Here's how the part is built. I have some questions about the finished solid (model axes, mm). Face numbers are marked on the shaded views. A direction names the side the tool comes from. Coordinates: 2 decimals unless noted, no trailing zeros. Write each loop counter-clockwise with the first axis right and the second up, starting at its lowest first coordinate (ties: lowest second). Pieces come first, ordered by that corner, then holes. Notation, with made-up numbers: (23, 27) - (56, 27) arc R17 cw to (56, 43) - close; hole circle Ø8 at (5, 9). An arc over 180 degrees is marked (long way). Answer in a Markdown table with one row per item. Add a question column.
Item 1: Imagine slicing it at C-C (z = 31). Please give me the cut outline in (x, y), plus the area to 3 significant figures.
Item 2: Which directions (+Z, -Z, +X, -X, +Y, -Y) give clear straight access to the entire face, cutting with the end or side of a thin tool? Please do the marked faces 1, 2 and 3.
Item 3: I'm going to push flat-ended pins straight in: pin 1 (3.5 mm diameter, centred on x = -5, z = -11, fed in from +Y); pin 2 (5 mm diameter, centred on y = 9, z = 11, fed in from -X); pin 3 (3.5 mm diameter, centred on x = -36, z = 48, fed in from +Y). Where does each tip first touch, or does it pass through?
Item 4: Imagine slicing it at A-A (x = -40.5). Please give me the cut outline in (y, z), plus the area to 3 significant figures.
Item 5: If I drill on probe 1 along Z at (x, y) = (-39.5, 8); probe 2 along X at (y, z) = (24.25, 37); probe 3 along X at (y, z) = (10.25, -45), over which ranges is the centre line in solid material (lowest first)? Write a range as from..to.
Item 6: We'd pull the mould along X, two halves only. Please class the marked faces 4, 5 and 6: +X half, -X half, draft (parallel to the pull), parting line (faces both ways), or undercut.
Item 7: Imagine slicing it at D-D (x = 47). Please give me the cut outline in (y, z), plus the area to 3 significant figures.
Item 8: Imagine slicing it at B-B (z = 46). Please give me the cut outline in (x, y), plus the area to 3 significant figures.
from build123d import *

# Parameters (mm, degrees)
BOSS_EXTRUDE1_DEPTH      = 2.5
BOSS_EXTRUDE1_DEPTH_BACK = 5
SKETCH3_W                = 7
SKETCH3_H                = 22
BOSS_EXTRUDE4_DEPTH      = 2.5
BOSS_EXTRUDE5_DEPTH      = 20
SKETCH7_R                = 3.75
BOSS_EXTRUDE6_DEPTH      = 5.5
SKETCH10_R               = 1.05
CUT_EXTRUDE1_DEPTH       = 2.5
SKETCH14_W               = 125
SKETCH14_H               = 7.5
SKETCH14_W_2             = 18
SKETCH14_H_2             = 1.5
BOSS_EXTRUDE8_DEPTH      = 10
SKETCH15_W               = 2.2
SKETCH15_H               = 17.5
SKETCH15_W_2             = 2.5
BOSS_EXTRUDE9_DEPTH      = 10
SKETCH16_R               = 1.4
CUT_EXTRUDE3_DEPTH       = 114
SKETCH17_W               = 7
SKETCH17_H               = 30
BOSS_EXTRUDE10_DEPTH     = 70
SKETCH18_W               = 45.75
SKETCH18_H               = 7.5
BOSS_EXTRUDE11_DEPTH     = 10


with BuildPart() as part:
    # Sketch2 → Boss-Extrude1 (new, two sides: drawn at the far end of the back side and taken through both)
    with BuildSketch(Plane(origin=(0, 0, 0), x_dir=(1, 0, 0), z_dir=(0, 1, 0)).offset(-BOSS_EXTRUDE1_DEPTH_BACK)):
        with BuildLine():
            Line((62.5, 25), (62.5, -25))
            ThreePointArc((62.5, -25), (53.127416998, -47.627416998), (30.5, -57))
            Line((30.5, -57), (23.5, -57))
            Line((23.5, -57), (23.5, -35))
            Line((23.5, -35), (30.5, -35))
            ThreePointArc((30.5, -35), (40.5, -25), (30.5, -15))
            Line((30.5, -15), (-38.5, -15))
            ThreePointArc((-38.5, -15), (-48.5, -25), (-38.5, -35))
            Line((-38.5, -35), (-31.5, -35))
            Line((-31.5, -35), (-31.5, -57))
            Line((-31.5, -57), (-38.5, -57))
            Line((-38.5, -57), (-62.5, -57))
            Line((-62.5, -57), (-62.5, 57))
            Line((-62.5, 57), (-38.5, 57))
            Line((-38.5, 57), (-31.5, 57))
            Line((-31.5, 57), (-31.5, 35))
            Line((-31.5, 35), (-38.5, 35))
            ThreePointArc((-38.5, 35), (-48.5, 25), (-38.5, 15))
            Line((-38.5, 15), (30.5, 15))
            ThreePointArc((30.5, 15), (40.5, 25), (30.5, 35))
            Line((30.5, 35), (23.5, 35))
            Line((23.5, 35), (23.5, 57))
            Line((23.5, 57), (30.5, 57))
            ThreePointArc((30.5, 57), (53.127416998, 47.627416998), (62.5, 25))
        make_face()
    extrude(amount=BOSS_EXTRUDE1_DEPTH + BOSS_EXTRUDE1_DEPTH_BACK)

    # Sketch3 → Boss-Extrude4 (add)
    with BuildSketch(Plane(origin=(0, 2.5, 0), x_dir=(1, 0, 0), z_dir=(0, 1, 0))):
        with Locations((-35, -46)):
            Rectangle(SKETCH3_W, SKETCH3_H)
        with Locations((27, -46)):
            Rectangle(SKETCH3_W, SKETCH3_H)
        with Locations((27, 46)):
            Rectangle(SKETCH3_W, SKETCH3_H)
        with Locations((-35, 46)):
            Rectangle(SKETCH3_W, SKETCH3_H)
    extrude(amount=BOSS_EXTRUDE4_DEPTH)

    # Sketch6 → Boss-Extrude5 (add)
    with BuildSketch(Plane(origin=(0, 5, 0), x_dir=(1, 0, 0), z_dir=(0, 1, 0))):
        Polygon((-38.5, -35), (-31.5, -35), (-31.5, -57), (-38.5, -57), (-38.5, -54.5), (-34, -54.5), (-34, -37.5), (-38.5, -37.5), align=None)
        Polygon((30.5, -35), (23.5, -35), (23.5, -57), (30.5, -57), (30.5, -54.5), (26, -54.5), (26, -37.5), (30.5, -37.5), align=None)
        Polygon((30.5, 37.5), (30.5, 35), (23.5, 35), (23.5, 57), (30.5, 57), (30.5, 54.5), (26, 54.5), (26, 37.5), align=None)
        Polygon((-38.5, 37.5), (-38.5, 35), (-31.5, 35), (-31.5, 57), (-38.5, 57), (-38.5, 54.5), (-34, 54.5), (-34, 37.5), align=None)
    extrude(amount=BOSS_EXTRUDE5_DEPTH)

    # Sketch7 → Boss-Extrude6 (add)
    with BuildSketch(Plane.ZY.offset(-23.5)):
        with Locations((46, 13.75)):
            Circle(SKETCH7_R)
        with Locations(Location((-46, 13.75, 0), (0, 0, 180))):
            Circle(SKETCH7_R)
    extrude(amount=BOSS_EXTRUDE6_DEPTH)

    # Sketch10 → Cut-Extrude1 (cut)
    with BuildSketch(Plane(origin=(-31.5, 0, 0), x_dir=(0, 0, -1), z_dir=(1, 0, 0))):
        with Locations((-42.5, 22)):
            Circle(SKETCH10_R)
        with Locations(Location((-49.5, 22, 0), (0, 0, 180))):
            Circle(SKETCH10_R)
        with Locations((-49.5, 8)):
            Circle(SKETCH10_R)
        with Locations(Location((-42.5, 8, 0), (0, 0, 180))):
            Circle(SKETCH10_R)
        with Locations((42.5, 8)):
            Circle(SKETCH10_R)
        with Locations(Location((49.5, 8, 0), (0, 0, 180))):
            Circle(SKETCH10_R)
        with Locations((49.5, 22)):
            Circle(SKETCH10_R)
        with Locations(Location((42.5, 22, 0), (0, 0, 180))):
            Circle(SKETCH10_R)
    extrude(amount=-CUT_EXTRUDE1_DEPTH, mode=Mode.SUBTRACT)

    # Sketch14 → Boss-Extrude8 (add)
    with BuildSketch(Plane(origin=(0, 2.5, 0), x_dir=(1, 0, 0), z_dir=(0, 1, 0))):
        Rectangle(SKETCH14_W, SKETCH14_H)
        Polygon((-56.5, -49.5), (-62.5, -49.5), (-62.5, -57), (-56.5, -57), (-56.5, -55.5), align=None)
        with Locations((-47.5, -56.25)):
            Rectangle(SKETCH14_W_2, SKETCH14_H_2)
        Polygon((-62.5, 57), (-62.5, 49.5), (-56.5, 49.5), (-56.5, 55.5), (-56.5, 57), align=None)
        with Locations((-47.5, 56.25)):
            Rectangle(SKETCH14_W_2, SKETCH14_H_2)
    extrude(amount=BOSS_EXTRUDE8_DEPTH)

    # Sketch15 → Boss-Extrude9 (add)
    with BuildSketch(Plane.ZY.offset(62.5)):
        with Locations((0, 3.75)):
            Rectangle(SKETCH15_W, SKETCH15_H)
        with Locations((55.75, 3.75)):
            Rectangle(SKETCH15_W_2, SKETCH15_H)
        with Locations((50.75, 3.75)):
            Rectangle(SKETCH15_W_2, SKETCH15_H)
        with Locations((-50.75, 3.75)):
            Rectangle(SKETCH15_W_2, SKETCH15_H)
        with Locations((-55.75, 3.75)):
            Rectangle(SKETCH15_W_2, SKETCH15_H)
    extrude(amount=BOSS_EXTRUDE9_DEPTH)

    # Sketch16 → Cut-Extrude3 (cut)
    with BuildSketch(Plane.XY.offset(57)):
        with Locations((-67.5, 7.25)):
            Circle(SKETCH16_R)
        with Locations((-67.5, 0.25)):
            Circle(SKETCH16_R)
    extrude(amount=-CUT_EXTRUDE3_DEPTH, mode=Mode.SUBTRACT)

    # Sketch17 → Boss-Extrude10 (add)
    with BuildSketch(Plane.XY.offset(-35)):
        with Locations((-35, 10)):
            Rectangle(SKETCH17_W, SKETCH17_H)
        with Locations((27, 10)):
            Rectangle(SKETCH17_W, SKETCH17_H)
    extrude(amount=BOSS_EXTRUDE10_DEPTH)

    # Sketch18 → Boss-Extrude11 (add)
    with BuildSketch(Plane.ZY.offset(62.5)):
        with Locations((-26.625, -1.25)):
            Rectangle(SKETCH18_W, SKETCH18_H)
        with Locations((26.625, -1.25)):
            Rectangle(SKETCH18_W, SKETCH18_H)
    extrude(amount=BOSS_EXTRUDE11_DEPTH)


solid = part.part
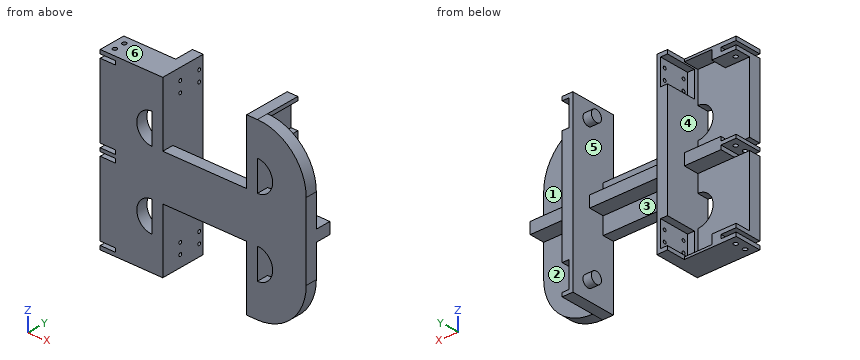
Here are the results:
| question | item | result |
|---|---|---|
| 1 | outline | (-72.5, -5) - (-46.5, -5) - (-46.5, 2.5) - (-72.5, 2.5) - close; (-38.5, -5) - (-31.5, -5) - (-31.5, 25) - (-38.5, 25) - close; (23.5, -5) - (30.5, -5) - (30.5, 25) - (23.5, 25) - close; (38.5, -5) - (61.93, -5) - (61.93, 2.5) - (38.5, 2.5) - close |
| 1 | area | 791 mm2 |
| 2 | face 1 | +Z, +X, +Y |
| 2 | face 2 | -Z, +X, +Y |
| 2 | face 3 | -Z, +Y |
| 3 | pin 1 | stops at y = 2.5 |
| 3 | pin 2 | stops at x = -38.5 |
| 3 | pin 3 | stops at y = 5 |
| 4 | outline | (-5, -57) - (12.5, -57) - (12.5, -55.5) - (2.5, -55.5) - (2.5, -34.8) - (-5, -34.8) - close; (-5, -15.2) - (2.5, -15.2) - (2.5, -3.75) - (12.5, -3.75) - (12.5, 3.75) - (2.5, 3.75) - (2.5, 15.2) - (-5, 15.2) - close; (-5, 34.8) - (2.5, 34.8) - (2.5, 55.5) - (12.5, 55.5) - (12.5, 57) - (-5, 57) - close |
| 4 | area | 666 mm2 |
| 5 | probe 1 | z = -57..-55.5, -3.75..3.75, 55.5..57 |
| 5 | probe 2 | x = -38.5..-31.5, 23.5..30.5 |
| 5 | probe 3 | x = -34..-31.5, 18..26 |
| 6 | face 4 | undercut |
| 6 | face 5 | undercut |
| 6 | face 6 | draft |
| 7 | outline | (-5, -52.42) - (2.5, -52.42) - (2.5, -3.75) - (12.5, -3.75) - (12.5, 3.75) - (2.5, 3.75) - (2.5, 52.42) - (-5, 52.42) - close |
| 7 | area | 861 mm2 |
| 8 | outline | (-72.5, -5) - (-31.5, -5) - (-31.5, 25) - (-34, 25) - (-34, 5) - (-38.5, 5) - (-38.5, 2.5) - (-72.5, 2.5) - close; (18, 10) - (23.5, 10) - (23.5, -5) - (54.65, -5) - (54.65, 2.5) - (30.5, 2.5) - (30.5, 5) - (26, 5) - (26, 25) - (23.5, 25) - (23.5, 17.5) - (18, 17.5) - close |
| 8 | area | 717 mm2 |
